The model under review builds one solid part; all positions refer to its coordinate system, in mm. Coordinates: 2 decimals unless noted, no trailing zeros. Loops run counter-clockwise (first coordinate to the right, second up) from the corner with the lowest first, then second, coordinate; pieces in that order, holes last. Notation, with made-up numbers: M -3,-30 L 6,-30 A12 cw 6,-22 Z; hole C 32.25,-28.75 d5. An arc over 180 degrees is marked long. One line per item, written item: value.
```python
from build123d import *

# Parameters (mm, degrees)
F0_W     = 3
F0_H     = 2.55
F1_DEPTH = 4.25
F3_DEPTH = 0.5
F4_R     = 0.2


with BuildPart() as f1:
    # F0 (on Front) → F1 (new body, symmetric)
    with BuildSketch(Plane.XZ):
        with Locations((0, 1.275)):
            Rectangle(F0_W, F0_H)
    extrude(amount=F1_DEPTH, both=True)

    # F2 (on Right) → F3 (join, symmetric)
    with BuildSketch(Plane.YZ):
        with BuildLine():
            Line((-4.260209, 0.09), (-4.260209, 0.89))
            Line((-4.260209, 0.89), (-4.460209, 0.89))
            Line((-4.460209, 0.89), (-4.460209, 0.09))
            ThreePointArc((-4.460209, 0.09), (-4.372341, -0.122132), (-4.160209, -0.21))
            Line((-4.160209, -0.21), (-2.425445, -0.21))
            Line((-2.425445, -0.21), (-2.425445, -0.01))
            Line((-2.425445, -0.01), (-4.160209, -0.01))
            ThreePointArc((-4.160209, -0.01), (-4.23092, 0.019289), (-4.260209, 0.09))
        make_face()
        with BuildLine():
            Line((4.460209, 0.09), (4.460209, 0.89))
            Line((4.460209, 0.89), (4.260209, 0.89))
            Line((4.260209, 0.89), (4.260209, 0.09))
            ThreePointArc((4.260209, 0.09), (4.23092, 0.019289), (4.160209, -0.01))
            Line((4.160209, -0.01), (2.425445, -0.01))
            Line((2.425445, -0.01), (2.425445, -0.21))
            Line((2.425445, -0.21), (4.160209, -0.21))
            ThreePointArc((4.160209, -0.21), (4.372341, -0.122132), (4.460209, 0.09))
        make_face()
    extrude(amount=F3_DEPTH, both=True)

    # F4
    f4_edges = [f1.edges().sort_by_distance(p)[0] for p in [
        (1.5, 4.25, 1.275),
        (1.5, 0, 2.55),
        (1.5, -4.25, 1.275),
        (1.5, 0, 0),
        (-1.5, 0, 2.55),
        (-1.5, 4.25, 1.275),
        (-1.5, 0, 0),
        (-1.5, -4.25, 1.275),
        (0, 4.25, 2.55),
        (0, -4.25, 2.55),
    ]]
    fillet(f4_edges, radius=F4_R)


solid = f1.part
```
(1) Add section A-A on y = 3.5. State the section outline as (x, z) points, then the cut area to 3 significant figures.
Checks:
outline: M -1.5,0.2 A0.2 ccw -1.3,0 L 1.3,0 A0.2 ccw 1.5,0.2 L 1.5,2.35 A0.2 ccw 1.3,2.55 L -1.3,2.55 A0.2 ccw -1.5,2.35 Z; M -0.5,-0.21 L 0.5,-0.21 L 0.5,-0.01 L -0.5,-0.01 Z
area: 7.82 mm^2
(2) Add section D-D on y = -0.5. State the section outline as (x, z) points.
Checks:
outline: M -1.5,0.2 A0.2 ccw -1.3,0 L 1.3,0 A0.2 ccw 1.5,0.2 L 1.5,2.35 A0.2 ccw 1.3,2.55 L -1.3,2.55 A0.2 ccw -1.5,2.35 Z
(3) Add section C-C on x = 0.4. State the section outline as (y, z) points.
Checks:
outline: M -4.46,0.09 A0.3 ccw -4.16,-0.21 L -2.43,-0.21 L -2.43,-0.01 L -4.16,-0.01 A0.1 cw -4.2,0 L 4.2,0 A0.1 cw 4.16,-0.01 L 2.43,-0.01 L 2.43,-0.21 L 4.16,-0.21 A0.3 ccw 4.46,0.09 L 4.46,0.89 L 4.26,0.89 L 4.26,0.09 A0.1 cw 4.25,0.05 L 4.25,2.35 A0.2 ccw 4.05,2.55 L -4.05,2.55 A0.2 ccw -4.25,2.35 L -4.25,0.05 A0.1 cw -4.26,0.09 L -4.26,0.89 L -4.46,0.89 Z
(4) To check wall thickness, follow L1, parallel to Y at x = 0.1, z = 1.5; L2, parallel to Z at x = 0.75, y = 0.5. State the ranges of each line that lie inside material, in increasing order. Write a range as [from, to].
Checks:
L1: [-4.25, 4.25]
L2: [0, 2.55]
(5) Draft analysis for pull direction Y (two halves, no side actions). For faces 1 (the face through (0, 3, -0.21)), 2 (the face through (0, 0, 0)), state which applies: pulls with the +Y half, pulls with the -Y half, needs draft (parallel to the pull), parting line crosses it, or undercut.
Checks:
face 1: needs draft
face 2: undercut
(6) Add section B-B on z = 0.6. State the section outline as (x, y) points, then the cut area to 3 significant figures.
Checks:
outline: M -1.5,-4.05 A0.2 ccw -1.3,-4.25 L 1.3,-4.25 A0.2 ccw 1.5,-4.05 L 1.5,4.05 A0.2 ccw 1.3,4.25 L -1.3,4.25 A0.2 ccw -1.5,4.05 Z; M -0.5,-4.46 L 0.5,-4.46 L 0.5,-4.26 L -0.5,-4.26 Z; M -0.5,4.26 L 0.5,4.26 L 0.5,4.46 L -0.5,4.46 Z
area: 25.9 mm^2
